```python
from build123d import *

# Parameters (mm, degrees)
F0_R     = 18.5
F1_DEPTH = 250
F0_R_2   = 21
F2_DEPTH = 158
F3_SIZE  = 2
F5_R     = 5
F6_DEPTH = 50


with BuildPart() as f1:
    # F0 (on Right) → F1 (new body, symmetric)
    with BuildSketch(Plane.YZ):
        Circle(F0_R)
    extrude(amount=F1_DEPTH, both=True)

    # F0 (on Right) → F2 (join, symmetric)
    with BuildSketch(Plane.YZ):
        Circle(F0_R_2)
        Circle(F0_R, mode=Mode.SUBTRACT)
    extrude(amount=F2_DEPTH, both=True)

    # F3
    f3_edges = [f1.edges().sort_by_distance(p)[0] for p in [
        (250, -18.5, 0),
        (-250, -18.5, 0),
    ]]
    chamfer(f3_edges, length=F3_SIZE)

    # F5 (on face) → F6 (cut, symmetric)
    with BuildSketch(Plane.XZ):
        with Locations((-198, 0)):
            Circle(F5_R)
        with Locations((198, 0)):
            Circle(F5_R)
    extrude(amount=F6_DEPTH, both=True, mode=Mode.SUBTRACT)


solid = f1.part
```
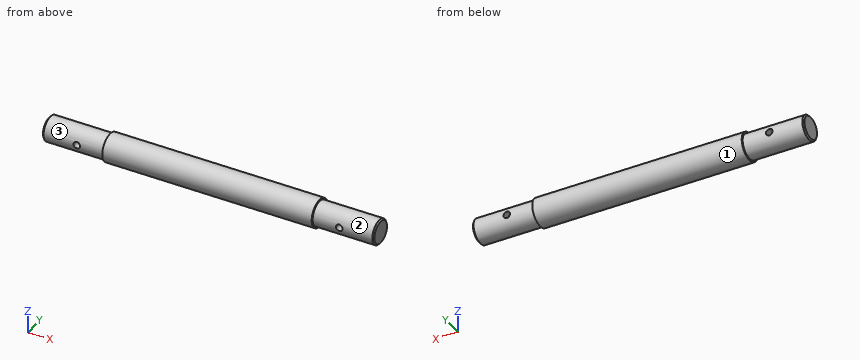
Read the model definition and answer for the solid it produces. Units are mm, in the model's axes. Face numbers are marked on the shaded views. A direction names the side the tool comes from. Give positions to 0.01 mm unless a question says otherwise; leave off trailing zeros. Write each loop counter-clockwise with the first axis right and the second up, starting at its lowest first coordinate (ties: lowest second). Pieces come first, ordered by that corner, then holes. Notation, with made-up numbers: M -12,39.25 L 4,39.25 A15 ccw 4,52.25 Z; hole C -37.75,61 d7. An arc over 180 degrees is marked long. Put each result on its own line as item: value. Start each with the question number.
1. Which of the six approach directions +Z, -Z, +X, -X, +Y, -Y give full straight-line access (tool end or side, diameter ignored) to the marked faces 1, 2 and 3?
2. Consider line 1 along X through (y, z) = (-8, 0); line 2 along X through (y, z) = (-3, -3); line 3 along X through (y, z) = (18.5, -7). Determine where each line is inside the solid, lowest interval first.
3. The part is cut by section A-A, the plane z = 0. Give the vertices of the cut face in (x, y).
4. Each of these flat-tipped pins is pushed along its axis until it touches: pin 1 Ø11.5 at (x, z) = (198, 0) entering from -Y; pin 2 Ø12 at (x, z) = (-103, -16.5) entering from -Y; pin 3 Ø16 at (x, z) = (-198, 0) entering from +Y. Where does it stop, or does it pass through?
5. The part is cut by section C-C, the plane x = -12.5. Give the vertices of the cut face in (y, z).
6. The part is cut by section D-D, the plane x = 198. Give the vertices of the cut face in (y, z), and give its area (3 significant figures).
7. The part is cut by section B-B, the plane y = 0. Give the vertices of the cut face in (x, z), and give its area (3 significant figures).
Final values:
1. face 1: +X, -X
1. face 2: +X
1. face 3: -X
2. line 1: x = -250 to -203, -193 to 193, 203 to 250
2. line 2: x = -250 to -202, -194 to 194, 202 to 250
2. line 3: x = -158 to 158
3. outline: M -250,-16.5 L -248,-18.5 L -203,-18.5 L -203,18.5 L -248,18.5 L -250,16.5 Z; M -193,-18.5 L -158,-18.5 L -158,-21 L 158,-21 L 158,-18.5 L 193,-18.5 L 193,18.5 L 158,18.5 L 158,21 L -158,21 L -158,18.5 L -193,18.5 Z; M 203,-18.5 L 248,-18.5 L 250,-16.5 L 250,16.5 L 248,18.5 L 203,18.5 Z
4. pin 1: stops at y = -18.5
4. pin 2: stops at y = -18.19
4. pin 3: stops at y = 18.5
5. outline: C 0,0 d42
6. outline: M -17.81,-5 A18.5 ccw 17.81,-5 Z; M -17.81,5 L 17.81,5 A18.5 ccw Z
6. area: 710 mm²
7. outline: M -250,-16.5 L -248,-18.5 L -158,-18.5 L -158,-21 L 158,-21 L 158,-18.5 L 248,-18.5 L 250,-16.5 L 250,16.5 L 248,18.5 L 158,18.5 L 158,21 L -158,21 L -158,18.5 L -248,18.5 L -250,16.5 Z; hole C -198,0 d10; hole C 198,0 d10
7. area: 19,900 mm²
